Read the model definition and answer for the solid it produces. Units are mm, in the model's axes. Round coordinates to 2 decimals unless told otherwise and drop trailing zeros. Order: outer loops, then holes, each group sorted by start corner. A loop starts at its lowest first (then second) coordinate and runs counter-clockwise, first axis right, second up. Notation, with made-up numbers: (34.5, 9.25) - (53.5, 9.25) arc R32 ccw to (53.5, 44.25) - close; hole circle Ø3 at (34.25, -8). An arc over 180 degrees is marked (long way). Answer as a JSON object with one key per item and string values. Group by question number.
Q1. Consider line 1 (Y direction, x = 41.5, z = -51.5); line 2 (X direction, y = 49, z = -39.5); line 3 (X direction, y = 20, z = -7). Determine where each line is inside the solid, lowest interval first.
Q2. A cutting plane is placed at D-D on x = 118.5. Determine the outline of the cut face in (y, z), and give its area (3 significant figures).
Q3. A cutting plane is placed at C-C on y = 42. Determine the outline of the cut face in (x, z).
Q4. Given pin 1 Ø5 at (x, z) = (157, -16.5) entering from -Y; pin 2 Ø6 at (x, y) = (65.5, 111) entering from -Z; pin 3 Ø5 at (x, z) = (84.5, -48.5) entering from +Y; pin 4 Ø3 at (x, z) = (124.5, -35) entering from +Y, each flat-ended and moving along its own axis, determine where each tip first touches the part or whether it passes through.
Q5. A cutting plane is placed at A-A on x = 163.5. Determine the outline of the cut face in (y, z), and give its area (3 significant figures).
Q6. A cutting plane is placed at B-B on z = -10.5. Determine the outline of the cut face in (x, y).
```python
from build123d import *

# Parameters (mm, degrees)
BOSS_EXTRUDE1_DEPTH = 203.2
SKETCH2_W           = 344.402501539
SKETCH2_H           = 780.457540957
CUT_EXTRUDE1_DEPTH  = 59.371664787


with BuildPart() as part:
    # Sketch1 → Boss-Extrude1 (new body)
    with BuildSketch(Plane(origin=(0, 0, 0), x_dir=(0, 0, -1), z_dir=(1, 0, 0))):
        with BuildLine():
            Line((0, 0), (31.75, 0))
            ThreePointArc((31.75, 0), (54.200640303, 9.299359697), (63.5, 31.75))
            Line((63.5, 31.75), (63.5, 95.25))
            ThreePointArc((63.5, 95.25), (54.200640303, 117.700640303), (31.75, 127))
            Line((31.75, 127), (0, 127))
            Line((0, 127), (-19.05, 127))
            Line((-19.05, 127), (-19.05, 0))
            Line((-19.05, 0), (0, 0))
        make_face()
    extrude(amount=BOSS_EXTRUDE1_DEPTH)

    # Sketch2 → Cut-Extrude1 (cut, through all)
    with BuildSketch(Plane(origin=(69.85, 0, 69.85), x_dir=(0, 1, 0), z_dir=(0.707106781, 0, 0.707106781))):
        with Locations((32.995160032, -188.585378543)):
            Rectangle(SKETCH2_W, SKETCH2_H)
    extrude(amount=CUT_EXTRUDE1_DEPTH, mode=Mode.SUBTRACT)


solid = part.part
```
Result set:
{
 "1": {"line 1": "y = 6.89 to 120.11", "line 2": "x = 0 to 179.2", "line 3": "x = 0 to 146.7"},
 "2": {"outline": "(0, -31.75) arc R31.75 ccw to (31.75, -63.5) - (95.25, -63.5) arc R31.75 ccw to (127, -31.75) - (127, 19.05) - (0, 19.05) - close", "area": "10,100 mm²"},
 "3": {"outline": "(0, -63.5) - (203.2, -63.5) - (120.65, 19.05) - (0, 19.05) - close"},
 "4": {"pin 1": "stops at y = 0", "pin 2": "stops at z = -60.83", "pin 3": "stops at y = 123.62", "pin 4": "stops at y = 126.95"},
 "5": {"outline": "(0, -31.75) arc R31.75 ccw to (31.75, -63.5) - (95.25, -63.5) arc R31.75 ccw to (127, -31.75) - (127, -23.8) - (0, -23.8) - close", "area": "4,610 mm²"},
 "6": {"outline": "(0, 0) - (150.2, 0) - (150.2, 127) - (0, 127) - close"}
}
